The model under review builds one solid part; all positions refer to its coordinate system, in mm. A direction names the side the tool comes from. Coordinates: 2 decimals unless noted, no trailing zeros. Order: outer loops, then holes, each group sorted by start corner. A loop starts at its lowest first (then second) coordinate and runs counter-clockwise, first axis right, second up. Notation, with made-up numbers: M 89,42 L 93,42 A21 ccw 93,70 Z; hole C 22.5,75 d5. An arc over 180 degrees is marked long. One line per item, written item: value.
Autodesk Inventor part; units mm, degrees
ref_plane "YZ Plane" through (0, 0, 0) normal (1, 0, 0) x (0, 1, 0)
ref_plane "XZ Plane" through (0, 0, 0) normal (0, 1, 0) x (-1, 0, 0)
ref_plane "XY Plane" through (0, 0, 0) normal (0, 0, 1) x (1, 0, 0)
sketch "Sketch1" plane through (0, 0, 0) normal (0, 1, 0) x (-1, 0, 0)
  line L0 (-5, 5) -> (5, 5) construction
  line L1 (5, 5) -> (5, -5) construction
  line L2 (5, -5) -> (-5, -5) construction
  line L3 (-5, -5) -> (-5, 5) construction
  line L4 (-5, 5) -> (5, -5) construction
  line L5 (5, 5) -> (-5, -5) construction
  line L6 (6.5, 22.5) -> (-6.5, 22.5)
  line L7 (-6.5, 22.5) -> (-6.5, -22.5)
  line L8 (-6.5, -22.5) -> (6.5, -22.5)
  line L9 (6.5, 22.5) -> (-6.5, -22.5) construction
  line L10 (-6.5, 22.5) -> (6.5, -22.5) construction
  arc A0 (6.5, -22.5) -> (6.5, 22.5) centre (-13.3431, 0) ccw
  point P0 (0, 0)
  dimension "d0" = 10
  dimension "d1" = 10
  dimension "d2" = 13
  dimension "d3" = 45
  dimension "d4" = 30
extrude "Extrusion1" add sketch "Sketch1" along normal blind 10
sketch "Sketch2" plane through (0, 0, 0) normal (0, -1, 0) x (1, 0, 0)
  line L0 (-5, 5) -> (5, 5)
  line L1 (5, 5) -> (5, -5)
  line L2 (5, -5) -> (-5, -5)
  line L3 (-5, -5) -> (-5, 5)
  line L4 (-5, 5) -> (5, -5) construction
  line L5 (5, 5) -> (-5, -5) construction
  point P0 (0, 0)
  dimension "d7" = 10
  dimension "d8" = 10
extrude "Extrusion2" add sketch "Sketch2" along normal blind 20
properties part number "holder"
(1) We need section D-D, the plane x = -6. State the section outline as (y, z) points, plus the area to 3 significant figures.
Geometry results:
outline: M 0,-22.5 L 10,-22.5 L 10,22.5 L 0,22.5 Z
area: 450 mm2
(2) For L1, parallel to Y at x = -2.75, z = 9.5; L2, parallel to Z at x = 2, y = -0.25, list the stretches that pass through material, from the lowest coordinate up.
Geometry results:
L1: y = 0 to 10
L2: z = -5 to 5
(3) Insertion check: pin 1 Ø2 at (x, y) = (-0.5, -16) entering from -Z; pin 2 Ø10 at (x, z) = (-5, 15.5) entering from -Y; pin 3 Ø5 at (x, y) = (1.5, -1.5) entering from +Z; pin 4 Ø8 at (y, z) = (-6, 1) entering from +X. Each pin has a flat end and moves straight along its axis. Give the tip position at first contact, or say it passes through.
Geometry results:
pin 1: stops at z = -5
pin 2: stops at y = 0
pin 3: stops at z = 22.5
pin 4: stops at x = 5
(4) We need section B-B, the plane y = -13.5. State the section outline as (x, z) points.
Geometry results:
outline: M -5,-5 L 5,-5 L 5,5 L -5,5 Z
(5) We need section A-A, the plane x = 2.75. State the section outline as (y, z) points, plus the area to 3 significant figures.
Geometry results:
outline: M -20,-5 L 0,-5 L 0,-22.5 L 10,-22.5 L 10,22.5 L 0,22.5 L 0,5 L -20,5 Z
area: 650 mm2
(6) Tool access review of faces 1 (the flat face through (0, 5, -22.5)), 2 (the flat face through (5, -10, 0)), 3 (the flat face through (0, -10, 5)), 4 (the flat face through (0, -10, -5)), 5 (the flat face through (-5, -10, 0)): name each direction out of +Z, -Z, +X, -X, +Y, -Y from which nothing blocks a thin tool from reaching the whole face with its end or side.
Geometry results:
face 1: -Z, +X, -X, +Y, -Y
face 2: +Z, -Z, +X, -Y
face 3: +Z, +X, -X, -Y
face 4: -Z, +X, -X, -Y
face 5: +Z, -Z, -X, -Y
(7) We need section C-C, the plane z = 2. State the section outline as (x, y) points, plus the area to 3 significant figures.
Geometry results:
outline: M -16.59,0 L -5,0 L -5,-20 L 5,-20 L 5,0 L 6.5,0 L 6.5,10 L -16.59,10 Z
area: 431 mm2
